Can you work these out from the drawing? Everything is in mm from the part's minimum corner. Round coordinates to 2 decimals unless told otherwise and drop trailing zeros. Loops run counter-clockwise (first coordinate to the right, second up) from the corner with the lowest first, then second, coordinate; pieces in that order, holes last. Notation, with made-up numbers: M 83.25,66.25 L 137.25,66.25 A15 ccw 137.25,91.25 Z; hole C 62,-5.5 d3. An arc over 180 degrees is marked long. Use a Markdown table: item, result.
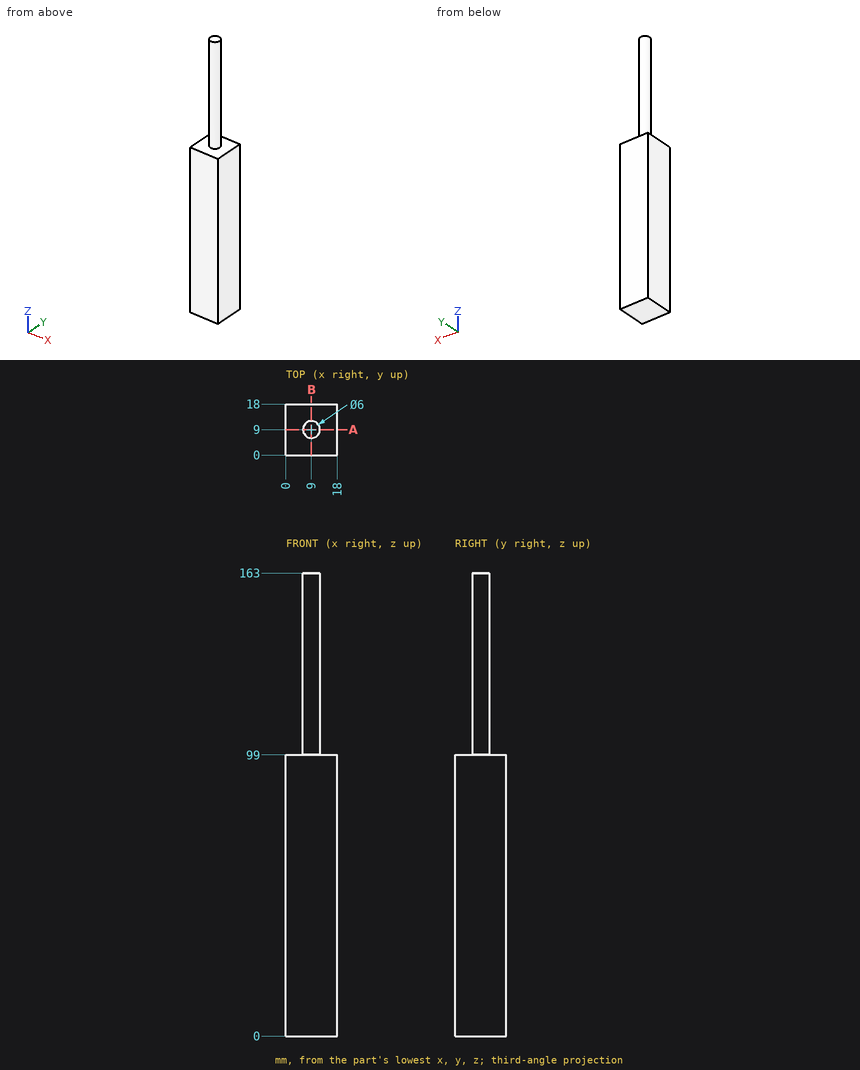
Q1. Will these pins go through, and if not, where does the flat tip stop? P1, Ø3, axis at x = 3, y = 15.5, coming from the -Z side; P2, Ø4, axis at x = 13, y = 5.5, coming from the +Z side; P3, Ø10, axis at x = 5.5, z = 108.5, coming from the +Y side.
Return value:
| item | result |
|---|---|
| P1 | stops at z = 0 |
| P2 | stops at z = 99 |
| P3 | stops at y = 12 |
Q2. Imagine slicing it at A-A, the plane y = 9. Please give me the cut outline in (x, z), then the cut area to 3 significant figures.
Return value:
| item | result |
|---|---|
| outline | M 0,0 L 18,0 L 18,99 L 12,99 L 12,163 L 6,163 L 6,99 L 0,99 Z |
| area | 2,170 mm^2 |
Q3. I need wall thicknesses on line 1 (Z direction, x = 16, y = 4.5); line 2 (X direction, y = 10.75, z = 153). Which ranges of each line are inside material? Lowest first, please. Write a range as from..to.
Return value:
| item | result |
|---|---|
| line 1 | z = 0..99 |
| line 2 | x = 6.56..11.44 |
